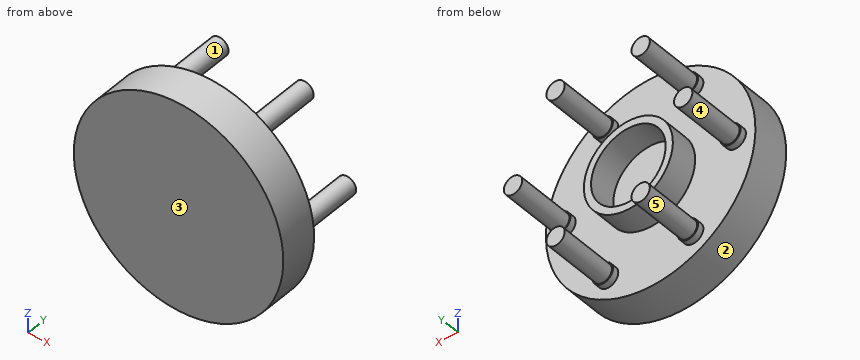
from build123d import *

# Parameters (mm, degrees)
SKETCH1_R           = 80
BOSS_EXTRUDE1_DEPTH = 29
SKETCH2_R           = 34
SKETCH2_R_2         = 28.5
BOSS_EXTRUDE2_DEPTH = 21
SKETCH3_R           = 7.75
BOSS_EXTRUDE3_DEPTH = 5
SKETCH4_R           = 7
BOSS_EXTRUDE4_DEPTH = 44.5


with BuildPart() as part:
    # Sketch1 → Boss-Extrude1 (new body)
    with BuildSketch(Plane(origin=(0, 0, 0), x_dir=(1, 0, 0), z_dir=(0, 1, 0))):
        with Locations(Location((0, 0, 0), (0, 0, 90))):
            Circle(SKETCH1_R)
    extrude(amount=BOSS_EXTRUDE1_DEPTH)

    # Sketch2 → Boss-Extrude2 (add)
    with BuildSketch(Plane(origin=(0, 29, 0), x_dir=(1, 0, 0), z_dir=(0, 1, 0))):
        with Locations(Location((0, 0, 0), (0, 0, 90))):
            Circle(SKETCH2_R)
        with Locations(Location((0, 0, 0), (0, 0, 90))):
            Circle(SKETCH2_R_2, mode=Mode.SUBTRACT)
    extrude(amount=BOSS_EXTRUDE2_DEPTH)

    # Sketch3 → Boss-Extrude3 (add)
    with BuildSketch(Plane(origin=(0, 29, 0), x_dir=(1, 0, 0), z_dir=(0, 1, 0))):
        with Locations(Location((65, 0, 0), (0, 0, 270))):
            Circle(SKETCH3_R)
        with Locations(Location((32.5, -56.291651246, 0), (0, 0, 270))):
            Circle(SKETCH3_R)
        with Locations(Location((-32.5, -56.291651246, 0), (0, 0, 270))):
            Circle(SKETCH3_R)
        with Locations(Location((-65, 0, 0), (0, 0, 270))):
            Circle(SKETCH3_R)
        with Locations(Location((-32.5, 56.291651246, 0), (0, 0, 270))):
            Circle(SKETCH3_R)
        with Locations(Location((32.5, 56.291651246, 0), (0, 0, 270))):
            Circle(SKETCH3_R)
    extrude(amount=BOSS_EXTRUDE3_DEPTH)

    # Sketch4 → Boss-Extrude4 (add)
    with BuildSketch(Plane(origin=(0, 34, 0), x_dir=(1, 0, 0), z_dir=(0, 1, 0))):
        with Locations(Location((65, 0, 0), (0, 0, 270))):
            Circle(SKETCH4_R)
        with Locations(Location((32.5, -56.291651246, 0), (0, 0, 270))):
            Circle(SKETCH4_R)
        with Locations(Location((-32.5, -56.291651246, 0), (0, 0, 270))):
            Circle(SKETCH4_R)
        with Locations(Location((-65, 0, 0), (0, 0, 270))):
            Circle(SKETCH4_R)
        with Locations(Location((-32.5, 56.291651246, 0), (0, 0, 270))):
            Circle(SKETCH4_R)
        with Locations(Location((32.5, 56.291651246, 0), (0, 0, 270))):
            Circle(SKETCH4_R)
    extrude(amount=BOSS_EXTRUDE4_DEPTH)


solid = part.part
Part model, mm, in its own coordinate system. Face numbers are marked on the shaded views. A direction names the side the tool comes from. Coordinates: 2 decimals unless noted, no trailing zeros. Loops run counter-clockwise (first coordinate to the right, second up) from the corner with the lowest first, then second, coordinate; pieces in that order, holes last. Notation, with made-up numbers: (71.25, -17) - (93.25, -17) arc R21 cw to (93.25, 21) - close; hole circle Ø2 at (-12, 67). An arc over 180 degrees is marked (long way). Write each question's results on one line, items separated by ' | '. Start each with the question number.
Q1. Drop flat-ended pins along their axis: pin 1 Ø12 at (y, z) = (31, 41) entering from +X; pin 2 Ø1.5 at (y, z) = (23.5, 52) entering from +X; pin 3 Ø8 at (x, y) = (-21, 53.5) entering from +Z; pin 4 Ø1 at (x, z) = (61.5, -22) entering from -Y. Give the stop position or say it passes through.
Q2. Slice it at A-A on y = 52. Give the cut face in (x, z), and give its area (3 significant figures).
Q3. Two-plate mould, pull along Z, no slides. Class the marked faces 3, 4 and 5: +Z half, -Z half, draft (parallel to the pull), parting line (faces both ways), or undercut.
Q4. Slice it at B-B on x = 0. Give the cut face in (y, z), and give its area (3 significant figures).
Q5. Slice it at D-D on y = 11. Give the cut face in (x, z).
Q6. Which spindle directions (+Z, -Z, +X, -X, +Y, -Y) get a long thin tool onto all of the face, cutting with end or side? Do the marked faces 1 and 2. Say none if no direction does.
Q7. Slice it at C-C on z = 0. Give the cut face in (x, y).
Q8. Probe line 1 along X through (y, z) = (39, 0); line 2 along Y through (x, z) = (67.5, 9.5); line 3 along Z through (x, y) = (-30.5, 60). List the from-to ranges inside material, lowest first.
Answer:
1) pin 1: stops at x = 71.77 | pin 2: stops at x = 61.43 | pin 3: stops at z = 28.15 | pin 4: stops at y = 0
2) outline: circle Ø14 at (-65, 0); circle Ø14 at (-32.5, -56.29); circle Ø14 at (-32.5, 56.29); circle Ø14 at (32.5, -56.29); circle Ø14 at (32.5, 56.29); circle Ø14 at (65, 0) | area: 924 mm2
3) face 3: draft | face 4: parting line | face 5: undercut
4) outline: (0, -80) - (29, -80) - (29, -34) - (50, -34) - (50, -28.5) - (29, -28.5) - (29, 28.5) - (50, 28.5) - (50, 34) - (29, 34) - (29, 80) - (0, 80) - close | area: 4,870 mm2
5) outline: circle Ø160 at (0, 0)
6) face 1: +Y | face 2: +Y, -Y
7) outline: (-80, 0) - (80, 0) - (80, 29) - (72.75, 29) - (72.75, 34) - (72, 34) - (72, 78.5) - (58, 78.5) - (58, 34) - (57.25, 34) - (57.25, 29) - (34, 29) - (34, 50) - (28.5, 50) - (28.5, 29) - (-28.5, 29) - (-28.5, 50) - (-34, 50) - (-34, 29) - (-57.25, 29) - (-57.25, 34) - (-58, 34) - (-58, 78.5) - (-72, 78.5) - (-72, 34) - (-72.75, 34) - (-72.75, 29) - (-80, 29) - close
8) line 1: x = -72 to -58, -34 to -28.5, 28.5 to 34, 58 to 72 | line 2: y = 0 to 29 | line 3: z = -63 to -49.58, 49.58 to 63
